Verification items for the finished model (mm, model axes). Face numbers are marked on the shaded views. Give positions to 0.01 mm unless a question says otherwise; leave off trailing zeros. Write each loop counter-clockwise with the first axis right and the second up, starting at its lowest first coordinate (ties: lowest second). Pieces come first, ordered by that corner, then holes. Notation, with made-up numbers: (-35.5, 72) -> (-4.5, 72) arc R23 ccw to (-4.5, 85) -> close; hole circle Ø6 at (52, -29). An arc over 180 degrees is marked (long way). Write item = value, one per line.
from build123d import *

# Parameters (mm, degrees)
SKETCH1_W           = 76.2
SKETCH1_H           = 50.8
BOSS_EXTRUDE1_DEPTH = 88.9
SKETCH2_R           = 5.25
CUT_EXTRUDE1_DEPTH  = 300
SKETCH3_W           = 76.2
SKETCH3_H           = 63.5
CUT_EXTRUDE2_DEPTH  = 5


with BuildPart() as part:
    # Sketch1 → Boss-Extrude1 (new body)
    with BuildSketch(Plane(origin=(0, 0, 0), x_dir=(1, 0, 0), z_dir=(0, 1, 0))):
        with Locations((38.1, 25.4)):
            Rectangle(SKETCH1_W, SKETCH1_H)
    extrude(amount=BOSS_EXTRUDE1_DEPTH)

    # Sketch2 → Cut-Extrude1 (cut)
    with BuildSketch(Plane.XY):
        with Locations((38.1, 57.15)):
            Circle(SKETCH2_R)
    extrude(amount=-CUT_EXTRUDE1_DEPTH, mode=Mode.SUBTRACT)

    # Sketch3 → Cut-Extrude2 (cut)
    with BuildSketch(Plane.XY):
        with Locations((38.1, 57.15)):
            Rectangle(SKETCH3_W, SKETCH3_H)
    extrude(amount=-CUT_EXTRUDE2_DEPTH, mode=Mode.SUBTRACT)


solid = part.part
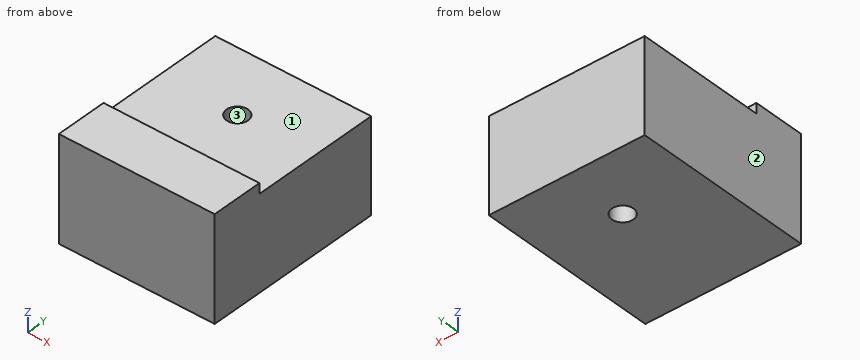
Item 1: Sectioned sample at C-C on x = 16. Record the cut outline in (y, z).
Response values:
outline = (0, -50.8) -> (88.9, -50.8) -> (88.9, -5) -> (25.4, -5) -> (25.4, 0) -> (0, 0) -> close
Item 2: Sectioned sample at D-D on y = 34. Record the cut outline in (x, z).
Response values:
outline = (0, -50.8) -> (76.2, -50.8) -> (76.2, -5) -> (0, -5) -> close
Item 3: Go/stop test with flat-tipped pins: P1, Ø1.5, axis at x = 51.5, z = -3.5, coming from the +Y side; P2, Ø12, axis at x = 38.1, y = 57.15, coming from the +Z side. Record where each tip stops, or that it passes through.
Response values:
P1 = 25.4
P2 = -5
Item 4: Sectioned sample at A-A on x = 38.1. Record the cut outline in (y, z).
Response values:
outline = (0, -50.8) -> (51.9, -50.8) -> (51.9, -5) -> (25.4, -5) -> (25.4, 0) -> (0, 0) -> close; (62.4, -50.8) -> (88.9, -50.8) -> (88.9, -5) -> (62.4, -5) -> close
Item 5: Material ranges on line 1 (Y direction, x = 38.1, z = -35.5); line 2 (X direction, y = 57, z = -14); line 3 (Z direction, x = 20.5, y = 35.5), recorded low to high.
Response values:
line_1 = 0 to 51.9, 62.4 to 88.9
line_2 = 0 to 32.85, 43.35 to 76.2
line_3 = -50.8 to -5
Item 6: Mould release check, pull along X, two halves, no side actions. Record for the marked faces 1, 2 and 3: +X half, -X half, draft (parallel to the pull), parting line (faces both ways), or undercut.
Response values:
face_1 = draft
face_2 = -X half
face_3 = undercut
Item 7: Sectioned sample at B-B on y = 55.5. Record the cut outline in (x, z).
Response values:
outline = (0, -50.8) -> (33.12, -50.8) -> (33.12, -5) -> (0, -5) -> close; (43.08, -50.8) -> (76.2, -50.8) -> (76.2, -5) -> (43.08, -5) -> close
